from build123d import *

# Parameters (mm, degrees)
CROQUIS1_W              = 36.7
CROQUIS1_H              = 40
CROQUIS1_R              = 4
SALIENTE_EXTRUIR1_DEPTH = 7
CHAFL_N1_SIZE           = 1
CROQUIS3_R              = 6.55
CORTAR_EXTRUIR1_DEPTH   = 2
CROQUIS5_W              = 36.7
CROQUIS5_H              = 7
CORTAR_EXTRUIR2_DEPTH   = 51.36836805
CROQUIS6_R              = 7
SALIENTE_EXTRUIR2_DEPTH = 2
SALIENTE_EXTRUIR3_START = 2
CROQUIS7_R              = 7
SALIENTE_EXTRUIR3_DEPTH = 2
SALIENTE_EXTRUIR4_DEPTH = 2


with BuildPart() as part:
    # Croquis1 → Saliente-Extruir1 (new body)
    with BuildSketch(Plane(origin=(0, 0, 0), x_dir=(1, 0, 0), z_dir=(0, 1, 0))):
        Rectangle(CROQUIS1_W, CROQUIS1_H)
        with Locations(Location((0, 0, 0), (0, 0, 270))):
            Circle(CROQUIS1_R, mode=Mode.SUBTRACT)
    extrude(amount=SALIENTE_EXTRUIR1_DEPTH)

    # Croquis2 → Revolución1 (revolve)
    with BuildSketch(Plane(origin=(0, 0, 0), x_dir=(0, 0, -1), z_dir=(1, 0, 0))):
        Polygon((7, 7), (7, 12), (5.5, 12), (5.5, 15), (7, 15), (7, 18), (5.5, 18), (5.5, 21), (7, 22.5), (7, 24.5), (4, 24.5), (4, 7), align=None)
    revolve(axis=Axis((0, 7, 0), (0, 1, 0)))

    # Chaflán1
    chafl_n1_edges = [part.edges().sort_by_distance(p)[0] for p in [
        (0, 12, 7),
        (0, 15, 7),
    ]]
    chamfer(chafl_n1_edges, length=CHAFL_N1_SIZE)

    # Croquis3 → Cortar-Extruir1 (cut)
    with BuildSketch(Plane.XZ):
        with Locations(Location((0, 0, 0), (0, 0, 270))):
            Circle(CROQUIS3_R)
    extrude(amount=-CORTAR_EXTRUIR1_DEPTH, mode=Mode.SUBTRACT)

    # Croquis5 → Cortar-Extruir2 (cut, through all)
    with BuildSketch(Plane.XY.offset(20)):
        with Locations((0, 3.5)):
            Rectangle(CROQUIS5_W, CROQUIS5_H)
    extrude(amount=-CORTAR_EXTRUIR2_DEPTH, mode=Mode.SUBTRACT)

    # Croquis6 → Saliente-Extruir2 (add)
    with BuildSketch(Plane.XZ.offset(-7)):
        with Locations(Location((0, 0, 0), (0, 0, 270))):
            Circle(CROQUIS6_R)
    extrude(amount=SALIENTE_EXTRUIR2_DEPTH)

    # Croquis7 → Saliente-Extruir3 (add)
    with BuildSketch(Plane(origin=(0, 24.5, 0), x_dir=(1, 0, 0), z_dir=(0, 1, 0)).offset(SALIENTE_EXTRUIR3_START)):
        with Locations(Location((0, 0, 0), (0, 0, 90))):
            Circle(CROQUIS7_R)
    extrude(amount=-SALIENTE_EXTRUIR3_DEPTH)

    # Croquis8 → Saliente-Extruir4 (add, symmetric)
    with BuildSketch(Plane(origin=(0, 0, 0), x_dir=(0, 0, -1), z_dir=(1, 0, 0))):
        with BuildLine():
            Line((-2.645751311, 5), (-5.196152423, 5))
            ThreePointArc((-5.196152423, 5), (0, -4), (5.196152423, 5))
            Line((5.196152423, 5), (2.645751311, 5))
            ThreePointArc((2.645751311, 5), (0, -2), (-2.645751311, 5))
        make_face()
    extrude(amount=SALIENTE_EXTRUIR4_DEPTH, both=True)


solid = part.part
Geometry check sheet. Reference: the model listing, model coordinates, mm. A direction names the side the tool comes from. Coordinates: 2 decimals unless noted, no trailing zeros. Order: outer loops, then holes, each group sorted by start corner. A loop starts at its lowest first (then second) coordinate and runs counter-clockwise, first axis right, second up. Notation, with made-up numbers: (26, 35) - (52, 35) arc R28 ccw to (52, 70) - close; hole circle Ø7 at (-1.5, -22). An arc over 180 degrees is marked (long way). One line per item, written item: value.
(1) Sectioned sample at A-A (y = 2). Enter the section's corners in (x, z), and give its area (3 significant figures).
Data:
outline: (-2, -6) - (2, -6) - (2, -4) - (-2, -4) - close; (-2, 4) - (2, 4) - (2, 6) - (-2, 6) - close
area: 16.0 mm^2
(2) Thickness scan on probe 1 along Y at (x, z) = (0.05, 0); probe 2 along X at (y, z) = (17.25, 0); probe 3 along Y at (x, z) = (5, 4.25). Record the ranges inside material, lowest first. Write a range as from..to.
Data:
probe 1: y = -4..-2, 5..7, 24.5..26.5
probe 2: x = -7..-4, 4..7
probe 3: y = 5..11.44, 15.56..18, 22.06..26.5
(3) Depth check by flat-ended pin: pin 1 Ø7 at (y, z) = (-1, 2) entering from +X; pin 2 Ø4.5 at (y, z) = (0, 1.5) entering from -X; pin 3 Ø1 at (x, y) = (-2, 6) entering from +Z. Enter the tip coordinate at first touch or a pass-through.
Data:
pin 1: stops at x = 2
pin 2: stops at x = -2
pin 3: stops at z = 6.84
(4) Release check for a two-part mould opening along Z. For faces 1 (the face through (0, 26.5, 0)), 2 (the face through (0, 24.5, 0)), 3 (the face through (2.681, 17.014, -6.466)), 4 (the face through (3.905, 15.628, 0.867)) record: +Z half, -Z half, draft (parallel to the pull), parting line (faces both ways), or undercut.
Data:
face 1: draft
face 2: undercut
face 3: parting line
face 4: undercut
(5) Sectioned sample at B-B (x = 0). Count the separate pieces of the cut face and the enclosed holes in it, and give its area (3 significant figures).
Data:
separate pieces: 1
enclosed holes: 2
area: 183 mm^2
(6) Access from +Z, -Z, +X, -X, +Y, -Y to the whole of each face (thin tool, end or side, straight path). Record for faces 5 (the face through (0, -2, 0)), 6 (the face through (-2, -2.4, 0.1)), 7 (the face through (2, -2.4, 0.1)), 8 (the face through (5.37, 13.52, 1.19)).
Data:
face 5: +X, -X
face 6: +Z, -Z, -X, -Y
face 7: +Z, -Z, +X, -Y
face 8: none
